Source: CAD feature listing. Evaluate the final solid. Frame: model axes, mm. Face numbers are marked on the shaded views. A direction names the side the tool comes from. Round coordinates to 2 decimals unless told otherwise and drop trailing zeros. Order: outer loops, then holes, each group sorted by start corner. A loop starts at its lowest first (then second) coordinate and runs counter-clockwise, first axis right, second up. Notation, with made-up numbers: (78.25, 39) -> (104.25, 39) arc R21 cw to (104.25, 43) -> close; hole circle Ø5 at (74, 56.25). An arc over 180 degrees is marked (long way). Answer as CSV lines item,"result".
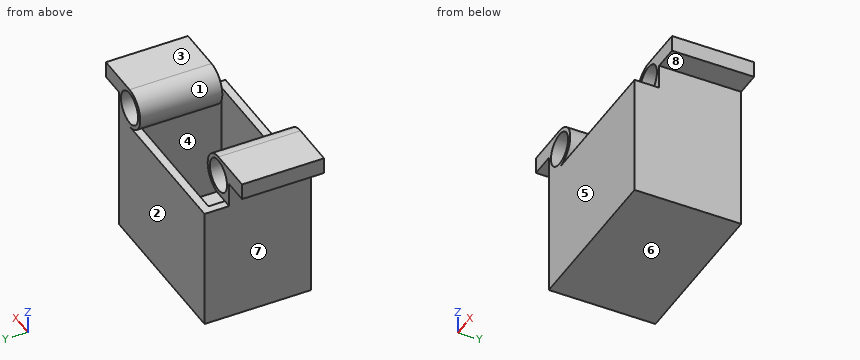
from build123d import *

# Parameters (mm, degrees)
SKETCH_1_W          = 20
SKETCH_1_H          = 13
EXTRUDE_1_DEPTH     = 15
SHELL_1_T           = -1
SKETCH_2_R          = 2.5
SKETCH_2_R_2        = 2
EXTRUDE_4_DEPTH     = 10
SKETCH_3_R          = 4.9
CUT_EXTRUDE_1_DEPTH = 0.2
SKETCH_9_R          = 2.5
SKETCH_9_R_2        = 2
EXTRUDE_8_DEPTH     = 10
SKETCH_6_W          = 2
SKETCH_6_H          = 10
EXTRUDE_10_DEPTH    = 3
SKETCH_10_W         = 2
SKETCH_10_H         = 10
EXTRUDE_11_DEPTH    = 3


with BuildPart() as part:
    # Sketch 1 → Extrude 1 (new body)
    with BuildSketch(Plane.XY):
        Rectangle(SKETCH_1_W, SKETCH_1_H)
    extrude(amount=EXTRUDE_1_DEPTH)

    # Shell 1
    shell_1_openings = [part.faces().sort_by_distance(p)[0] for p in [
        (0, 0, 15),
    ]]
    offset(amount=SHELL_1_T, openings=shell_1_openings, kind=Kind.INTERSECTION)

    # Sketch 3 → Cut-Extrude 1 (cut)
    with BuildSketch(Plane.XY.offset(1)):
        with BuildLine():
            Line((4.9, 4.9), (2.1e-08, 4.9))
            ThreePointArc((2.1e-08, 4.9), (3.464823235, 3.46482322), (4.9, 0))
            Line((4.9, 0), (4.9, 4.9))
        make_face()
        with BuildLine():
            Line((2.1e-08, 4.9), (-4.9, 4.9))
            Line((-4.9, 4.9), (-4.9, 7e-09))
            ThreePointArc((-4.9, 7e-09), (-3.464823218, 3.464823238), (2.1e-08, 4.9))
        make_face()
        Circle(SKETCH_3_R)
        with BuildLine():
            ThreePointArc((0, -4.9), (-3.46482323, -3.464823225), (-4.9, 7e-09))
            Line((-4.9, 7e-09), (-4.9, -4.9))
            Line((-4.9, -4.9), (0, -4.9))
        make_face()
        with BuildLine():
            Line((4.9, -4.9), (4.9, 0))
            ThreePointArc((4.9, 0), (3.464823228, -3.464823228), (0, -4.9))
            Line((0, -4.9), (4.9, -4.9))
        make_face()
    extrude(amount=-CUT_EXTRUDE_1_DEPTH, mode=Mode.SUBTRACT)

    # Sketch 9 → Extrude 8 (add)
    # profile 1 of 3: a face of its own
    with BuildSketch(Plane(origin=(0, 6.5, 0), x_dir=(1, 0, 0), z_dir=(0, 1, 0))):
        with BuildLine():
            Line((10, -17.5), (10, -15))
            Line((10, -15), (7.5, -15))
            ThreePointArc((7.5, -15), (9.267766953, -15.732233047), (10, -17.5))
        make_face()
    # profile 2 of 3: a face of its own
    with BuildSketch(Plane(origin=(0, 6.5, 0), x_dir=(1, 0, 0), z_dir=(0, 1, 0))):
        with BuildLine():
            Line((10, -20), (10, -17.5))
            ThreePointArc((10, -17.5), (9.267766953, -19.267766953), (7.5, -20))
            Line((7.5, -20), (10, -20))
        make_face()
    # profile 3 of 3: a face of its own
    with BuildSketch(Plane(origin=(0, 6.5, 0), x_dir=(1, 0, 0), z_dir=(0, 1, 0))):
        with Locations((7.5, -17.5)):
            Circle(SKETCH_9_R)
        with Locations(Location((7.5, -17.5, 0), (0, 0, 270))):
            Circle(SKETCH_9_R_2, mode=Mode.SUBTRACT)
    extrude(amount=-EXTRUDE_8_DEPTH)


with BuildPart() as body_2:
    # Sketch 2 → Extrude 4 (new body)
    # profile 1 of 3: a face of its own
    with BuildSketch(Plane(origin=(0, 3.5, 0), x_dir=(1, 0, 0), z_dir=(0, 1, 0))):
        with BuildLine():
            ThreePointArc((-7.5, -20), (-9.267766953, -19.267766953), (-10, -17.5))
            Line((-10, -17.5), (-10, -20))
            Line((-10, -20), (-7.5, -20))
        make_face()
    # profile 2 of 3: a face of its own
    with BuildSketch(Plane(origin=(0, 3.5, 0), x_dir=(1, 0, 0), z_dir=(0, 1, 0))):
        with Locations((-7.5, -17.5)):
            Circle(SKETCH_2_R)
        with Locations(Location((-7.5, -17.5, 0), (0, 0, 270))):
            Circle(SKETCH_2_R_2, mode=Mode.SUBTRACT)
    # profile 3 of 3: a face of its own
    with BuildSketch(Plane(origin=(0, 3.5, 0), x_dir=(1, 0, 0), z_dir=(0, 1, 0))):
        with BuildLine():
            Line((-7.5, -15), (-10, -15))
            Line((-10, -15), (-10, -17.5))
            ThreePointArc((-10, -17.5), (-9.267766953, -15.732233047), (-7.5, -15))
        make_face()
    extrude(amount=-EXTRUDE_4_DEPTH)


    add(part.part)  # Extrude 10 merges part
    # Sketch 6 → Extrude 10 (add)
    with BuildSketch(Plane.ZY.offset(10)):
        with Locations((19, -1.5)):
            Rectangle(SKETCH_6_W, SKETCH_6_H)
    extrude(amount=EXTRUDE_10_DEPTH)

    # Sketch 10 → Extrude 11 (add)
    with BuildSketch(Plane(origin=(10, 0, 0), x_dir=(0, 0, -1), z_dir=(1, 0, 0))):
        with Locations((-19, 1.5)):
            Rectangle(SKETCH_10_W, SKETCH_10_H)
    extrude(amount=EXTRUDE_11_DEPTH)


solid = body_2.part
1. Reachability of the marked faces 4, 5, 6, 7 and 8 from +Z, -Z, +X, -X, +Y, -Y: full face, straight path, thin tool, end or side. Return the list, or none.
Results below:
face 4,"none"
face 5,"+Z, -Z, +X, -X, -Y"
face 6,"-Z, +X, -X, +Y, -Y"
face 7,"-Z, -X, +Y, -Y"
face 8,"-Z, +X, +Y, -Y"
2. Mould query, pull axis Z, two halves, no side actions, for the marked faces 1, 2 and 3. Classes: released by +Z, released by -Z, zero draft, split by the parting line, or undercut.
Results below:
face 1,"undercut"
face 2,"zero draft"
face 3,"released by +Z"
3. Pin query (flat end, axial travel): pin 1 (4 mm diameter, centred on y = -1.5, z = 12.5, fed in from +X); pin 2 (0.9 mm diameter, centred on x = 11, y = 3, fed in from -Z); pin 3 (5 mm diameter, centred on y = -5, z = 14, fed in from -X). Return the tip coordinate at first contact, or that it passes through.
Results below:
pin 1,"x = 10"
pin 2,"z = 18"
pin 3,"x = -10"
4. Section query B-B on y = -0.75. Return loops of the section in (x, z), and give its area (3 significant figures).
Results below:
outline,"(-13, 18) -> (-10, 18) -> (-10, 0) -> (10, 0) -> (10, 18) -> (13, 18) -> (13, 20) -> (7.5, 20) arc R2.5 ccw to (7.5, 15) -> (9, 15) -> (9, 1) -> (4.9, 1) -> (4.9, 0.8) -> (-4.9, 0.8) -> (-4.9, 1) -> (-9, 1) -> (-9, 15) -> (-7.5, 15) arc R2.5 ccw to (-7.5, 20) -> (-13, 20) -> close; hole circle Ø4 at (-7.5, 17.5); hole circle Ø4 at (7.5, 17.5)"
area,"77.5 mm2"
5. Section query D-D on x = 3.5. Return loops of the section in (y, z), and give its area (3 significant figures).
Results below:
outline,"(-6.5, 0) -> (6.5, 0) -> (6.5, 15) -> (5.5, 15) -> (5.5, 1) -> (4.9, 1) -> (4.9, 0.8) -> (-4.9, 0.8) -> (-4.9, 1) -> (-5.5, 1) -> (-5.5, 15) -> (-6.5, 15) -> close"
area,"39.0 mm2"
6. Section query A-A on z = 17.5. Return loops of the section in (x, y).
Results below:
outline,"(-10, -6.5) -> (-9.5, -6.5) -> (-9.5, 3.5) -> (-10, 3.5) -> close; (-5.5, -6.5) -> (-5, -6.5) -> (-5, 3.5) -> (-5.5, 3.5) -> close; (5, -3.5) -> (5.5, -3.5) -> (5.5, 6.5) -> (5, 6.5) -> close; (9.5, -3.5) -> (10, -3.5) -> (10, 6.5) -> (9.5, 6.5) -> close"
7. Section query C-C on z = 5.75. Return loops of the section in (x, y).
Results below:
outline,"(-10, -6.5) -> (10, -6.5) -> (10, 6.5) -> (-10, 6.5) -> close; hole (-9, -5.5) -> (9, -5.5) -> (9, 5.5) -> (-9, 5.5) -> close"
8. Line query: L1, parallel to X at y = 2.25, z = 17.5; L2, parallel to Y at x = 2.5, z = 2; L3, parallel to X at y = -4.5, z = 14.5. Output: solid intervals per line, ascending. Write a range as [from, to].
Results below:
L1,"[-10, -9.5], [-5.5, -5], [5, 5.5], [9.5, 10]"
L2,"[-6.5, -5.5], [5.5, 6.5]"
L3,"[-10, -9], [9, 10]"
